```python
from build123d import *

# Parameters (mm, degrees)
SKETCH1_R           = 2.75
BOSS_EXTRUDE1_DEPTH = 6.35
SKETCH2_R           = 2.75
CUT_EXTRUDE1_DEPTH  = 6.35


with BuildPart() as part:
    # Sketch1 → Boss-Extrude1 (new body)
    with BuildSketch(Plane(origin=(0, 0, 0), x_dir=(1, 0, 0), z_dir=(0, 1, 0))):
        with BuildLine():
            Line((7, 90), (7, 0))
            ThreePointArc((7, 0), (0, -7), (-7, 0))
            Line((-7, 0), (-7, 90))
            ThreePointArc((-7, 90), (0, 97), (7, 90))
        make_face()
        with Locations((0, 90)):
            Circle(SKETCH1_R, mode=Mode.SUBTRACT)
        Circle(SKETCH1_R, mode=Mode.SUBTRACT)
    extrude(amount=BOSS_EXTRUDE1_DEPTH)

    # Sketch2 → Cut-Extrude1 (cut)
    with BuildSketch(Plane(origin=(0, 0, 0), x_dir=(1, 0, 0), z_dir=(0, 1, 0))):
        with Locations((0, 90)):
            Circle(SKETCH2_R)
        with Locations((0, 80)):
            Circle(SKETCH2_R)
        with Locations((0, 70)):
            Circle(SKETCH2_R)
        with Locations((0, 60)):
            Circle(SKETCH2_R)
        with Locations((0, 50)):
            Circle(SKETCH2_R)
    extrude(amount=CUT_EXTRUDE1_DEPTH, mode=Mode.SUBTRACT)


solid = part.part
```
Part model, mm, in its own coordinate system. Round coordinates to 2 decimals unless told otherwise and drop trailing zeros. Loops run counter-clockwise (first coordinate to the right, second up) from the corner with the lowest first, then second, coordinate; pieces in that order, holes last.
1. Slice it at D-D (x = -5.5). Give the cut face in (y, z).
Solutions:
outline: (0, -94.33) - (6.35, -94.33) - (6.35, 4.33) - (0, 4.33) - close
2. Slice it at C-C (y = 1.75). Give the cut face in (x, z).
Solutions:
outline: (-7, -90) arc R7 ccw to (7, -90) - (7, 0) arc R7 ccw to (-7, 0) - close; hole circle Ø5.5 at (0, -90); hole circle Ø5.5 at (0, -80); hole circle Ø5.5 at (0, -70); hole circle Ø5.5 at (0, -60); hole circle Ø5.5 at (0, -50); hole circle Ø5.5 at (0, 0)
3. Slice it at A-A (x = 0). Give the cut face in (y, z).
Solutions:
outline: (0, -97) - (6.35, -97) - (6.35, -92.75) - (0, -92.75) - close; (0, -87.25) - (6.35, -87.25) - (6.35, -82.75) - (0, -82.75) - close; (0, -77.25) - (6.35, -77.25) - (6.35, -72.75) - (0, -72.75) - close; (0, -67.25) - (6.35, -67.25) - (6.35, -62.75) - (0, -62.75) - close; (0, -57.25) - (6.35, -57.25) - (6.35, -52.75) - (0, -52.75) - close; (0, -47.25) - (6.35, -47.25) - (6.35, -2.75) - (0, -2.75) - close; (0, 2.75) - (6.35, 2.75) - (6.35, 7) - (0, 7) - close
4. Two-plate mould, pull along X, no slides. Class faces 1 (the face through (7, 3, -46)), 2 (the face through (0, 3, 7)), 3 (the face through (-0.358, 3.131, -62.727)): pulls with the +X half, pulls with the -X half, needs draft (parallel to the pull), parting line crosses it, or undercut.
Solutions:
face 1: pulls with the +X half
face 2: parting line crosses it
face 3: undercut
5. Slice it at B-B (z = -50). Give the cut face in (x, y), and give its area (3 significant figures).
Solutions:
outline: (-7, 0) - (-2.75, 0) - (-2.75, 6.35) - (-7, 6.35) - close; (2.75, 0) - (7, 0) - (7, 6.35) - (2.75, 6.35) - close
area: 54.0 mm2
6. Drill centre lines: line 1 along X through (y, z) = (4.5, 0); line 2 along X through (y, z) = (1.5, -82.5); line 3 along Z through (x, y) = (-4, 3.75). Where is each one in solid material? Low to high.
Solutions:
line 1: x = -7 to -2.75, 2.75 to 7
line 2: x = -7 to -1.15, 1.15 to 7
line 3: z = -95.74 to 5.74
7. Flat gauge pins, fed straight in: pin 1 (1 mm diameter, centred on x = 4.5, y = 4, fed in from +Z); pin 2 (2 mm diameter, centred on x = -3, y = 1.5, fed in from -Z). Where does each tip first touch, or does it go through?
Solutions:
pin 1: stops at z = 5.74
pin 2: stops at z = -96.71
